Geometry check sheet. Reference: the model listing, model coordinates, mm. A direction names the side the tool comes from. Give positions to 0.01 mm unless a question says otherwise; leave off trailing zeros. Write each loop counter-clockwise with the first axis right and the second up, starting at its lowest first coordinate (ties: lowest second). Pieces come first, ordered by that corner, then holes.
(1) Tool access check on faces 4 (the flat face through (10, 0.25, -11)), 5 (the cylindrical face through (-9.9, 1.2, -10.5)), 6 (the flat face through (-12.25, -1, 11)). Record the directions out of +Z, -Z, +X, -X, +Y, -Y that give a thin tool (end or side, any length) a straight path to the whole face; none if there is none.
(2) Cross-section at C-C (z = -9). Record the boundary of the cut face in (x, y).
(3) Cross-section at B-B (x = -15). Record the boundary of the cut face in (y, z).
(4) Thickness scan on line 1 along Z through (x, y) = (-15, -1.3); line 2 along Z through (x, y) = (-9, 1.85); line 3 along X through (y, z) = (0.15, 10). Record the ranges inside material, lowest first.
(5) Depth check by flat-ended pin: P1, Ø0.8, axis at y = -1, z = 12.5, coming from the -X side; P2, Ø5, axis at x = 8.5, z = 10.5, coming from the -Y side. Enter the tip coordinate at first touch or a pass-through.
(6) Cross-section at D-D (z = 10). Record the boundary of the cut face in (x, y).
(7) Cross-section at A-A (y = -0.15). Count the separate pieces of the cut face and the enclosed holes in it, and give its area (3 significant figures).
(8) Mould release check, pull along X, two halves, no side actions. Record for faces 1 (the flat face through (7.35, -1.02, 6.2)), 2 (the cylindrical face through (18.1, 0.03, 13.14)), 3 (the flat face through (-19, 0, 0)): +X half, -X half, draft (parallel to the pull), parting line (faces both ways), or undercut.
```python
from build123d import *

# Parameters (mm, degrees)
SKETCH_1_W              = 38
SKETCH_1_H              = 28
EXTRUDE_1_DEPTH         = 2.25
HOLE_WIZARD_3_5_3_5_2_D = 3.5
HOLE_WIZARD_3_5_3_5_4_D = 3.5
CUT_EXTRUDE_2_DEPTH     = 2.5
MIRROR_4_COPY_1_DEPTH   = 2.5
FILLET_2_R              = 3


with BuildPart() as part:
    # 草圖1 → 填料-伸長1 (new, symmetric)
    with BuildSketch(Plane(origin=(0, 0, 0), x_dir=(1, 0, 0), z_dir=(0, 1, 0))):
        Rectangle(SKETCH_1_W, SKETCH_1_H)
    extrude(amount=EXTRUDE_1_DEPTH, both=True)

    # Ø3.5 (3.5) 直徑孔2 (through all)
    with Locations(Plane(origin=(0, 2.25, 0), x_dir=(1, 0, 0), z_dir=(0, 1, 0))):
        with Locations((15, 10), (-15, -10), (-15, 10), (15, -10)):
            Hole(HOLE_WIZARD_3_5_3_5_2_D / 2)

    # Ø3.5 (3.5) 直徑孔4 (through all)
    with Locations(Plane(origin=(0, 2.25, 0), x_dir=(1, 0, 0), z_dir=(0, 1, 0))):
        with Locations((9, 9), (-9, -9), (-9, 9), (9, -9)):
            Hole(HOLE_WIZARD_3_5_3_5_4_D / 2)

    # 草圖9 → 除料-伸長2 (cut)
    with BuildSketch(Plane.XZ.offset(2.25)):
        Polygon((-12.25, 10.876388375), (-12.25, 14), (-5.75, 14), (-5.75, 10.876388375), (-5.75, 7.123611625), (-9, 5.24722325), (-12.25, 7.123611625), align=None)
    cut_extrude_2 = extrude(amount=-CUT_EXTRUDE_2_DEPTH, mode=Mode.SUBTRACT)

    # 鏡射3: 除料-伸長2 across plane
    add(cut_extrude_2.mirror(Plane.XY), mode=Mode.SUBTRACT)

    # 鏡射4: 除料-伸長2 across plane
    add(cut_extrude_2.mirror(Plane(origin=(0, 0, 0), x_dir=(0, 0, 1), z_dir=(1, 0, 0))), mode=Mode.SUBTRACT)

    # 鏡射4 copy 1 sketch → 鏡射4 copy 1 (cut)
    with BuildSketch(Plane(origin=(0, -2.25, 0), x_dir=(-1, 0, 0), z_dir=(0, -1, 0))):
        Polygon((-12.25, 10.876388375), (-12.25, 14), (-5.75, 14), (-5.75, 10.876388375), (-5.75, 7.123611625), (-9, 5.24722325), (-12.25, 7.123611625), align=None)
    extrude(amount=-MIRROR_4_COPY_1_DEPTH, mode=Mode.SUBTRACT)

    # 圓角2
    fillet_2_edges = [part.edges().sort_by_distance(p)[0] for p in [
        (19, 0, 14),
        (-19, 0, 14),
        (-19, 0, -14),
        (19, 0, -14),
    ]]
    fillet(fillet_2_edges, radius=FILLET_2_R)


solid = part.part
```
Reply:
1. face 4: -Z, -Y
1. face 5: +Y, -Y
1. face 6: +Z, -Y
2. outline: (-19, -2.25) - (-16.44, -2.25) - (-16.44, 2.25) - (-19, 2.25) - close; (-13.56, -2.25) - (-12.25, -2.25) - (-12.25, 0.25) - (-10.75, 0.25) - (-10.75, 2.25) - (-13.56, 2.25) - close; (-7.25, 0.25) - (-5.75, 0.25) - (-5.75, -2.25) - (5.75, -2.25) - (5.75, 0.25) - (7.25, 0.25) - (7.25, 2.25) - (-7.25, 2.25) - close; (10.75, 0.25) - (12.25, 0.25) - (12.25, -2.25) - (13.56, -2.25) - (13.56, 2.25) - (10.75, 2.25) - close; (16.44, -2.25) - (19, -2.25) - (19, 2.25) - (16.44, 2.25) - close
3. outline: (-2.25, -14) - (2.25, -14) - (2.25, -11.75) - (-2.25, -11.75) - close; (-2.25, -8.25) - (2.25, -8.25) - (2.25, 8.25) - (-2.25, 8.25) - close; (-2.25, 11.75) - (2.25, 11.75) - (2.25, 14) - (-2.25, 14) - close
4. line 1: z = -14 to -11.75, -8.25 to 8.25, 11.75 to 14
4. line 2: z = -14 to -10.75, -7.25 to 7.25, 10.75 to 14
4. line 3: x = -19 to -16.75, -13.25 to -12.25, -5.75 to 5.75, 12.25 to 13.25, 16.75 to 19
5. P1: stops at x = -18.79
5. P2: stops at y = 0.25
6. outline: (-19, -2.25) - (-16.75, -2.25) - (-16.75, 2.25) - (-19, 2.25) - close; (-13.25, -2.25) - (-12.25, -2.25) - (-12.25, 0.25) - (-10.44, 0.25) - (-10.44, 2.25) - (-13.25, 2.25) - close; (-7.56, 0.25) - (-5.75, 0.25) - (-5.75, -2.25) - (5.75, -2.25) - (5.75, 0.25) - (7.56, 0.25) - (7.56, 2.25) - (-7.56, 2.25) - close; (10.44, 0.25) - (12.25, 0.25) - (12.25, -2.25) - (13.25, -2.25) - (13.25, 2.25) - (10.44, 2.25) - close; (16.75, -2.25) - (19, -2.25) - (19, 2.25) - (16.75, 2.25) - close
7. separate pieces: 1
7. enclosed holes: 4
7. area: 815 mm2
8. face 1: undercut
8. face 2: +X half
8. face 3: -X half
